Part print with two shaded views. Sizes in mm from the minimum x, y, z corner. Coordinates: 2 decimals unless noted, no trailing zeros. Loops run counter-clockwise (first coordinate to the right, second up) from the corner with the lowest first, then second, coordinate; pieces in that order, holes last.
Item 1: Cut at C-C (x = 67.5). List the corners of the cut face in (y, z), and give its area (4 significant figures).
Item 2: Cut at D-D (x = 55). List the corners of the cut face in (y, z), and give its area (4 significant figures).
Item 3: Flat gauge pins, fed straight in: pin 1 (1.5 mm diameter, centred on y = 69, z = 2, fed in from +X); pin 2 (14 mm diameter, centred on x = 40.5, y = 54.5, fed in from +Z); pin 3 (1 mm diameter, centred on x = 11.5, z = 4.5, fed in from +Y). Where does each tip first touch, or does it go through?
Item 4: Cut at B-B (y = 44). List the corners of the cut face in (x, z), and give its area (4 significant figures).
Item 5: Cut at A-A (z = 6.5). List the corners of the cut face in (x, y).
Item 6: Drill centre lines: line 1 along Y through (x, z) = (29, 3.75); line 2 along X through (y, z) = (28, 7.25); line 3 along X through (y, z) = (50, 3.5). Where is each one in solid material? Low to high.
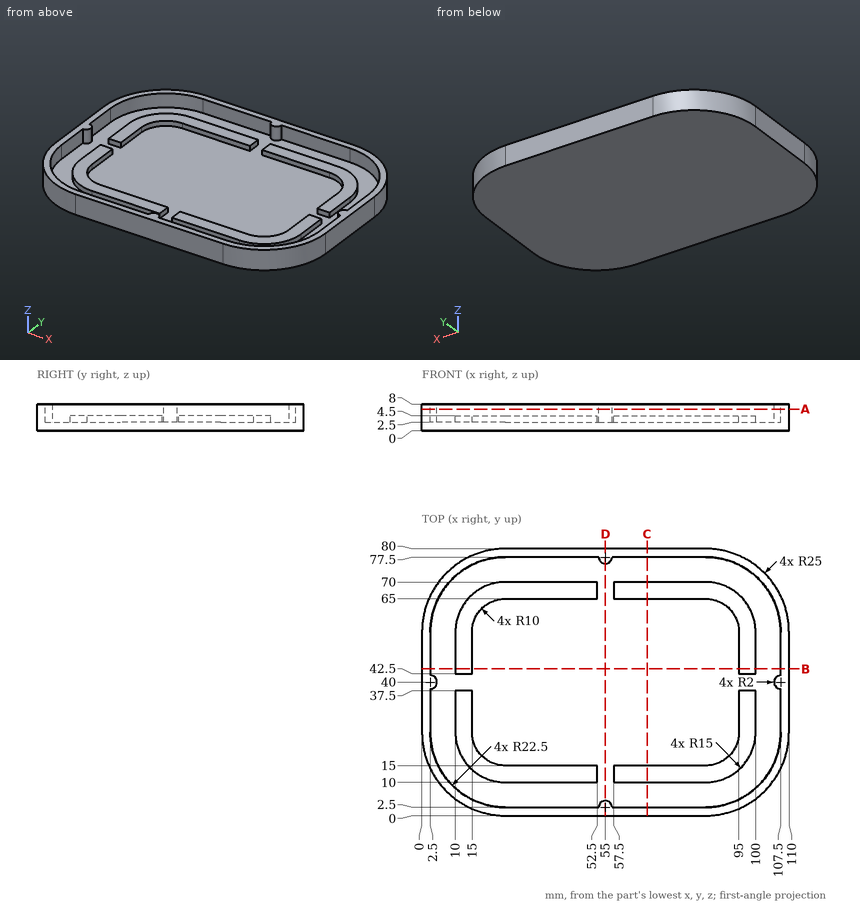
Filled sheet:
1. outline: (0, 0) - (80, 0) - (80, 8) - (77.5, 8) - (77.5, 2.5) - (70, 2.5) - (70, 4.5) - (65, 4.5) - (65, 2.5) - (15, 2.5) - (15, 4.5) - (10, 4.5) - (10, 2.5) - (2.5, 2.5) - (2.5, 8) - (0, 8) - close
1. area: 247.5 mm2
2. outline: (0, 0) - (80, 0) - (80, 8) - (75.5, 8) - (75.5, 2.5) - (4.5, 2.5) - (4.5, 8) - (0, 8) - close
2. area: 249.5 mm2
3. pin 1: stops at x = 106.2
3. pin 2: stops at z = 2.5
3. pin 3: stops at y = 76.35
4. outline: (0, 0) - (110, 0) - (110, 8) - (107.5, 8) - (107.5, 2.5) - (100, 2.5) - (100, 4.5) - (95, 4.5) - (95, 2.5) - (15, 2.5) - (15, 4.5) - (10, 4.5) - (10, 2.5) - (2.5, 2.5) - (2.5, 8) - (0, 8) - close
4. area: 322.5 mm2
5. outline: (0, 25) arc R25 ccw to (25, 0) - (85, 0) arc R25 ccw to (110, 25) - (110, 55) arc R25 ccw to (85, 80) - (25, 80) arc R25 ccw to (0, 55) - close; hole (2.5, 25) arc R22.5 ccw to (25, 2.5) - (53, 2.5) arc R2 cw to (57, 2.5) - (85, 2.5) arc R22.5 ccw to (107.5, 25) - (107.5, 38) arc R2 cw to (107.5, 42) - (107.5, 55) arc R22.5 ccw to (85, 77.5) - (57, 77.5) arc R2 cw to (53, 77.5) - (25, 77.5) arc R22.5 ccw to (2.5, 55) - (2.5, 42) arc R2 cw to (2.5, 38) - close
6. line 1: y = 0 to 2.5, 10 to 15, 65 to 70, 77.5 to 80
6. line 2: x = 0 to 2.5, 107.5 to 110
6. line 3: x = 0 to 2.5, 10 to 15, 95 to 100, 107.5 to 110
